Read the model definition and answer for the solid it produces. Units are mm, in the model's axes. Face numbers are marked on the shaded views. A direction names the side the tool comes from. Coordinates: 2 decimals unless noted, no trailing zeros. Write each loop counter-clockwise with the first axis right and the second up, starting at its lowest first coordinate (ties: lowest second). Pieces come first, ordered by that corner, then holes.
1) The part is cut by section C-C (y = 25). Determine the outline of the cut face in (x, z).
2) The part is cut by section A-A (x = 0). Determine the outline of the cut face in (y, z), then the cut area to 3 significant figures.
3) The part is cut by section B-B (z = 0). Determine the outline of the cut face in (x, y).
4) Find the intervals of material crossed by line 1 (Y direction, x = -22.5, z = 16.5); line 2 (Z direction, x = 0, y = 24.6), in increasing order.
5) Determine the mould class of the marked faces 1, 2 and 3 for opening direction X: +X half, -X half, draft (parallel to the pull), parting line (faces both ways), or undercut.
6) Which of the six approach directions +Z, -Z, +X, -X, +Y, -Y give full straight-line access (tool end or side, diameter ignored) to the marked faces 4, 5 and 6?
7) Each of these flat-tipped pins is pushed along its axis until it touches: pin 1 Ø1 at (x, y) = (-3.5, 21.5) entering from +Z; pin 2 Ø6 at (x, y) = (-22, 23.5) entering from -Z; pin 3 Ø11.5 at (x, z) = (0, 0) entering from +Y. Where does it stop, or does it pass through?
8) The part is cut by section D-D (z = -20). Determine the outline of the cut face in (x, y).
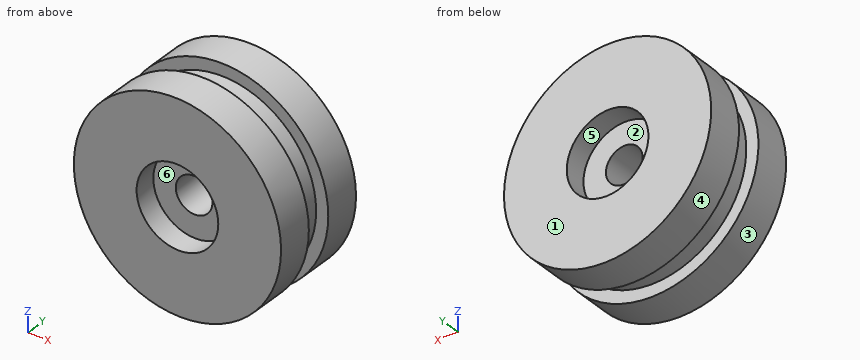
Autodesk Inventor part; units mm, degrees
ref_plane "YZ Plane" through (0, 0, 0) normal (1, 0, 0) x (0, 1, 0)
ref_plane "XZ Plane" through (0, 0, 0) normal (0, 1, 0) x (-1, 0, 0)
ref_plane "XY Plane" through (0, 0, 0) normal (0, 0, 1) x (1, 0, 0)
sketch "Sketch1" plane through (0, 0, 0) normal (0, 0, 1) x (1, 0, 0)
  line L0 (0, 0) -> (0, 20.9396) construction
  line L1 (5, 0) -> (28.3, 0)
  line L2 (28.3, 0) -> (28.3, 10)
  line L3 (28.3, 10) -> (25, 10)
  line L4 (25, 10) -> (25, 17)
  line L5 (25, 17) -> (28.3, 17)
  line L6 (28.3, 17) -> (28.3, 27)
  line L7 (28.3, 27) -> (5, 27)
  line L8 (5, 27) -> (5, 0)
  dimension "d1" = 3.3
  dimension "d2" = 7
  dimension "d4" = 10
  dimension "d15" = 25
  dimension "d16" = 5
revolve "Revolution1" add sketch "Sketch1" angle 360 about axis through (0, 0, 0) along (0, 1, 0)
sketch "Sketch2" plane through (0, 27, 0) normal (0, 1, 0) x (1, 0, 0)
  circle A0 centre (0, 0) radius 11.15
  dimension "d8" = 22.3
extrude "Extrusion1" cut sketch "Sketch2" against normal blind 6
sketch "Sketch3" plane through (0, 0, 0) normal (0, -1, 0) x (1, 0, 0)
  circle A0 centre (0, 0) radius 11.15
  dimension "d11" = 22.3
extrude "Extrusion2" cut sketch "Sketch3" against normal blind 6
properties part number "1213_Distal Roller_V1" material "Acetal Resin, White"
Reported:
1. outline: circle Ø56.6 at (0, 0); hole circle Ø22.3 at (0, 0)
2. outline: (0, -28.3) - (10, -28.3) - (10, -25) - (17, -25) - (17, -28.3) - (27, -28.3) - (27, -11.15) - (21, -11.15) - (21, -5) - (6, -5) - (6, -11.15) - (0, -11.15) - close; (0, 11.15) - (6, 11.15) - (6, 5) - (21, 5) - (21, 11.15) - (27, 11.15) - (27, 28.3) - (17, 28.3) - (17, 25) - (10, 25) - (10, 28.3) - (0, 28.3) - close
2. area: 1,060 mm2
3. outline: (-28.3, 0) - (-11.15, 0) - (-11.15, 6) - (-5, 6) - (-5, 21) - (-11.15, 21) - (-11.15, 27) - (-28.3, 27) - (-28.3, 17) - (-25, 17) - (-25, 10) - (-28.3, 10) - close; (5, 6) - (11.15, 6) - (11.15, 0) - (28.3, 0) - (28.3, 10) - (25, 10) - (25, 17) - (28.3, 17) - (28.3, 27) - (11.15, 27) - (11.15, 21) - (5, 21) - close
4. line 1: y = 0 to 10, 17 to 27
4. line 2: z = -28.3 to -11.15, 11.15 to 28.3
5. face 1: draft
5. face 2: undercut
5. face 3: parting line
6. face 4: +Y, -Y
6. face 5: +Y
6. face 6: -Y
7. pin 1: stops at z = 28.14
7. pin 2: stops at z = -20.97
7. pin 3: stops at y = 21
8. outline: (-20.02, 0) - (20.02, 0) - (20.02, 10) - (15, 10) - (15, 17) - (20.02, 17) - (20.02, 27) - (-20.02, 27) - (-20.02, 17) - (-15, 17) - (-15, 10) - (-20.02, 10) - close
